Geometry: final body of the model. Coordinates: model frame, mm. A direction names the side the tool comes from. Coordinates: 2 decimals unless noted, no trailing zeros. Write each loop counter-clockwise with the first axis right and the second up, starting at its lowest first coordinate (ties: lowest second). Pieces come first, ordered by that corner, then holes.
from build123d import *

# Parameters (mm, degrees)
SKETCH_R      = 50
EXTRUDE_DEPTH = 10


with BuildPart() as part:
    # Sketch → Extrude (new body)
    with BuildSketch(Plane.XY):
        Circle(SKETCH_R)
        Polygon((0, -36.217949), (-28.28525, 0), (-31.490379, 6.089741), (-31.490379, 10.897434), (-29.407051, 18.75), (-25.721149, 22.756409), (-21.554483, 25), (-12.419867, 23.557693), (-10.01602, 22.275639), (-6.330123, 18.26923), (-1.522433, 13.621796), (0, 11.538464), (3.605769, 15.865385), (6.810907, 20.673079), (9.054492, 22.756409), (12.900642, 26.762819), (15.945516, 27.724361), (21.23398, 27.724361), (26.682697, 23.397434), (28.926281, 18.589741), (29.246799, 15.224361), (29.246799, 11.538464), (28.445511, 7.692307), (27.804497, 4.326921), (25.240389, -1.121795), (21.394239, -4.967949), align=None, mode=Mode.SUBTRACT)
    extrude(amount=EXTRUDE_DEPTH)


solid = part.part
Item 1: Section A-A, the plane y = -26. Output: boundary loops of the cut face in (x, z), plus the area to 3 significant figures.
Derived:
outline: (-42.71, 0) - (-7.98, 0) - (-7.98, 10) - (-42.71, 10) - close; (7, 0) - (42.71, 0) - (42.71, 10) - (7, 10) - close
area: 704 mm2
Item 2: Section C-C, the plane x = -23. Output: boundary loops of the cut face in (y, z), plus the area to 3 significant figures.
Derived:
outline: (-44.4, 0) - (-6.77, 0) - (-6.77, 10) - (-44.4, 10) - close; (24.22, 0) - (44.4, 0) - (44.4, 10) - (24.22, 10) - close
area: 578 mm2
Item 3: Material intervals for probe 1 along X at (y, z) = (16.5, 4); probe 2 along Y at (x, z) = (7.5, 9.25); probe 3 along Y at (x, z) = (7, 1), sorted ascending.
Derived:
probe 1: x = -47.2 to -30, -4.5 to 4.03, 29.13 to 47.2
probe 2: y = -49.43 to -25.26, 21.31 to 49.43
probe 3: y = -49.51 to -25.99, 20.85 to 49.51
Item 4: Pull-direction query (X, two-part tool) for faces 1 (the flat face through (10, -22, 0)), 2 (the flat face through (23.34, -3.02, 4.93)); classes: released by +X, released by -X, zero draft, split by the parting line, or undercut.
Derived:
face 1: zero draft
face 2: undercut
Item 5: Pin query (flat end, axial travel): pin 1 (1.1 mm diameter, centred on y = 13, z = 4, fed in from -X); pin 2 (5 mm diameter, centred on y = -17.5, z = 7, fed in from -X); pin 3 (1.4 mm diameter, centred on y = 8.5, z = 6, fed in from +X). Return the tip coordinate at first contact, or that it passes through.
Derived:
pin 1: stops at x = -48.43
pin 2: stops at x = -47.7
pin 3: stops at x = 49.39
Item 6: Set-up query: faces 3 (the flat face through (10, -22, 10)), 4 (the flat face through (10.85, -20.37, 4.93)). Return all of +Z, -Z, +X, -X, +Y, -Y with unobstructed straight access to the full face (end or side cutting, diameter ignored); none if empty.
Derived:
face 3: +Z, +X, -X, +Y, -Y
face 4: +Z, -Z
Item 7: Section D-D, the plane x = 43. Output: boundary loops of the cut face in (y, z), plus the area to 3 significant figures.
Derived:
outline: (-25.51, 0) - (25.51, 0) - (25.51, 10) - (-25.51, 10) - close
area: 510 mm2
Item 8: Section B-B, the plane z = 7.75. Output: boundary loops of the cut face in (x, y), plus the area to 3 significant figures.
Derived:
outline: circle Ø100 at (0, 0); hole (-31.49, 6.09) - (-28.29, 0) - (0, -36.22) - (21.39, -4.97) - (25.24, -1.12) - (27.8, 4.33) - (28.45, 7.69) - (29.25, 11.54) - (29.25, 15.22) - (28.93, 18.59) - (26.68, 23.4) - (21.23, 27.72) - (15.95, 27.72) - (12.9, 26.76) - (9.05, 22.76) - (6.81, 20.67) - (3.61, 15.87) - (0, 11.54) - (-1.52, 13.62) - (-6.33, 18.27) - (-10.02, 22.28) - (-12.42, 23.56) - (-21.55, 25) - (-25.72, 22.76) - (-29.41, 18.75) - (-31.49, 10.9) - close
area: 5,590 mm2
